```python
from build123d import *

# Parameters (mm, degrees)
BOSS_EXTRUDE1_DEPTH = 10
SKETCH2_R           = 4.05
SKETCH2_R_2         = 1.975
CUT_EXTRUDE1_DEPTH  = 49.845189118
SKETCH14_W          = 50.25
SKETCH14_H          = 4.1
CUT_EXTRUDE13_DEPTH = 5
SKETCH16_W          = 4.6
SKETCH16_H          = 15
CUT_EXTRUDE15_DEPTH = 10
CUT_EXTRUDE14_DEPTH = 49.845189118
SKETCH19_W          = 7
SKETCH19_H          = 5
BOSS_EXTRUDE2_DEPTH = 1
CUT_EXTRUDE16_DEPTH = 8.95
FILLET1_R           = 0.5


with BuildPart() as part:
    # Sketch1 → Boss-Extrude1 (new body)
    with BuildSketch(Plane(origin=(0, 0, 0), x_dir=(1, 0, 0), z_dir=(0, 1, 0))):
        Polygon((-23, 23.2), (23, 23.2), (39.25, 23.2), (39.25, -23.2), (23, -23.2), (23, -27.3), (16, -27.3), (16, -23.2), (3.5, -23.2), (3.5, -27.3), (-3.5, -27.3), (-3.5, -23.2), (-16, -23.2), (-16, -27.3), (-23, -27.3), (-23, -23.2), (-27.25, -23.2), (-27.25, 23.2), align=None)
    extrude(amount=BOSS_EXTRUDE1_DEPTH)

    # Sketch2 → Cut-Extrude1 (cut, through all)
    with BuildSketch(Plane(origin=(0, 10, 0), x_dir=(1, 0, 0), z_dir=(0, 1, 0))):
        with Locations(Location((0, 0, 0), (0, 0, 270))):
            Circle(SKETCH2_R)
        with Locations(Location((-2.025, 15, 0), (0, 0, 270))):
            Circle(SKETCH2_R_2)
        with Locations(Location((-2.025, -15, 0), (0, 0, 270))):
            Circle(SKETCH2_R_2)
    extrude(amount=-CUT_EXTRUDE1_DEPTH, mode=Mode.SUBTRACT)

    # Sketch14 → Cut-Extrude13 (cut)
    with BuildSketch(Plane(origin=(0, 10, 0), x_dir=(1, 0, 0), z_dir=(0, 1, 0))):
        with Locations((-2.125, -25.25)):
            Rectangle(SKETCH14_W, SKETCH14_H)
    extrude(amount=-CUT_EXTRUDE13_DEPTH, mode=Mode.SUBTRACT)

    # Sketch16 → Cut-Extrude15 (cut)
    with BuildSketch(Plane.XZ):
        with Locations((34.45, 0)):
            Rectangle(SKETCH16_W, SKETCH16_H)
        with Locations((-22.45, 0)):
            Rectangle(SKETCH16_W, SKETCH16_H)
    extrude(amount=-CUT_EXTRUDE15_DEPTH, mode=Mode.SUBTRACT)

    # Sketch15 → Cut-Extrude14 (cut, through all)
    with BuildSketch(Plane(origin=(0, 10, 0), x_dir=(1, 0, 0), z_dir=(0, 1, 0))):
        with BuildLine():
            Line((13, -27.3), (13, -23.2))
            ThreePointArc((13, -23.2), (14.5, -21.7), (16, -23.2))
            Line((16, -23.2), (16, -27.3))
            ThreePointArc((16, -27.3), (14.5, -28.8), (13, -27.3))
        make_face()
        with BuildLine():
            Line((3.5, -27.3), (3.5, -23.2))
            ThreePointArc((3.5, -23.2), (5, -21.7), (6.5, -23.2))
            Line((6.5, -23.2), (6.5, -27.3))
            ThreePointArc((6.5, -27.3), (5, -28.8), (3.5, -27.3))
        make_face()
        with BuildLine():
            Line((-13, -27.3), (-13, -23.2))
            ThreePointArc((-13, -23.2), (-14.5, -21.7), (-16, -23.2))
            Line((-16, -23.2), (-16, -27.3))
            ThreePointArc((-16, -27.3), (-14.5, -28.8), (-13, -27.3))
        make_face()
        with BuildLine():
            Line((-3.5, -27.3), (-3.5, -23.2))
            ThreePointArc((-3.5, -23.2), (-5, -21.7), (-6.5, -23.2))
            Line((-6.5, -23.2), (-6.5, -27.3))
            ThreePointArc((-6.5, -27.3), (-5, -28.8), (-3.5, -27.3))
        make_face()
        with BuildLine():
            Line((23, -27.3), (23, -23.2))
            ThreePointArc((23, -23.2), (24.5, -21.7), (26, -23.2))
            Line((26, -23.2), (26, -27.3))
            ThreePointArc((26, -27.3), (24.5, -28.8), (23, -27.3))
        make_face()
        with BuildLine():
            Line((-23, -27.3), (-23, -23.2))
            ThreePointArc((-23, -23.2), (-24.5, -21.7), (-26, -23.2))
            Line((-26, -23.2), (-26, -27.3))
            ThreePointArc((-26, -27.3), (-24.5, -28.8), (-23, -27.3))
        make_face()
        with BuildLine():
            ThreePointArc((34.45, 7.284346805), (31.710660172, 6.439339828), (34.45, 5.594332852))
            ThreePointArc((34.45, 5.594332852), (37.189339828, 6.439339828), (34.45, 7.284346805))
        make_face()
        with BuildLine():
            ThreePointArc((34.45, -7.284346805), (31.710660172, -6.439339828), (34.45, -5.594332852))
            ThreePointArc((34.45, -5.594332852), (37.189339828, -6.439339828), (34.45, -7.284346805))
        make_face()
        with BuildLine():
            ThreePointArc((-22.45, -7.284346805), (-19.710660172, -6.439339828), (-22.45, -5.594332852))
            ThreePointArc((-22.45, -5.594332852), (-25.189339828, -6.439339828), (-22.45, -7.284346805))
        make_face()
        with BuildLine():
            ThreePointArc((-22.45, 7.284346805), (-25.189339828, 6.439339828), (-22.45, 5.594332852))
            ThreePointArc((-22.45, 5.594332852), (-19.710660172, 6.439339828), (-22.45, 7.284346805))
        make_face()
    extrude(amount=-CUT_EXTRUDE14_DEPTH, mode=Mode.SUBTRACT)

    # Sketch19 → Boss-Extrude2 (add)
    with BuildSketch(Plane(origin=(0, 0, -23.2), x_dir=(-1, 0, 0), z_dir=(0, 0, -1))):
        with Locations((-23.83, 2.5)):
            Rectangle(SKETCH19_W, SKETCH19_H)
    extrude(amount=BOSS_EXTRUDE2_DEPTH)

    # Sketch17 → Cut-Extrude16 (cut)
    with BuildSketch(Plane(origin=(0, 10, 0), x_dir=(1, 0, 0), z_dir=(0, 1, 0))):
        with BuildLine():
            Line((25.48, 24.2), (25.48, 15.85))
            ThreePointArc((25.48, 15.85), (23.83, 14.2), (22.18, 15.85))
            Line((22.18, 15.85), (22.18, 24.2))
            ThreePointArc((22.18, 24.2), (23.83, 25.85), (25.48, 24.2))
        make_face()
        with BuildLine():
            Line((1.65, -18.95), (1.65, -27.3))
            ThreePointArc((1.65, -27.3), (0, -28.95), (-1.65, -27.3))
            Line((-1.65, -27.3), (-1.65, -18.95))
            ThreePointArc((-1.65, -18.95), (0, -17.3), (1.65, -18.95))
        make_face()
    extrude(amount=-CUT_EXTRUDE16_DEPTH, mode=Mode.SUBTRACT)

    # Fillet1
    fillet1_edges = [part.edges().sort_by_distance(p)[0] for p in [
        (-27.25, 5, 23.2),
        (-27.25, 5, -23.2),
        (39.25, 5, -23.2),
        (39.25, 5, 23.2),
        (20.33, 2.5, -24.2),
        (27.33, 2.5, -24.2),
        (25.48, 3.025, -24.2),
        (22.18, 3.025, -24.2),
        (-1.65, 3.025, 27.3),
        (1.65, 3.025, 27.3),
        (-16, 2.5, 27.3),
        (-23, 2.5, 27.3),
        (23, 2.5, 27.3),
        (16, 2.5, 27.3),
        (3.5, 2.5, 27.3),
        (-3.5, 2.5, 27.3),
    ]]
    fillet(fillet1_edges, radius=FILLET1_R)


solid = part.part
```
Geometry check sheet. Reference: the model listing, model coordinates, mm. A direction names the side the tool comes from. Coordinates: 2 decimals unless noted, no trailing zeros. Order: outer loops, then holes, each group sorted by start corner. A loop starts at its lowest first (then second) coordinate and runs counter-clockwise, first axis right, second up. Notation, with made-up numbers: M -37,75.5 L -10,75.5 A11 cw -10,89.5 Z; hole C 40,37 d7. An arc over 180 degrees is marked long. Answer as a JSON object with one key per item and string values.
Q1. Cross-section at C-C on x = -5. Record the cut outline in (y, z), and give its area (3 significant figures).
Results are:
{"outline": "M 0,-23.2 L 10,-23.2 L 10,21.7 L 0,21.7 Z", "area": "449 mm²"}
Q2. Depth check by flat-ended pin: pin 1 Ø1.2 at (x, z) = (19, 24.5) entering from +Y; pin 2 Ø2.5 at (x, y) = (19.5, 7.5) entering from +Z; pin 3 Ø3 at (x, z) = (1.5, 10.5) entering from -Y; pin 4 Ø3 at (x, y) = (-2, 5) entering from -Z. Enter the tip coordinate at first touch or a pass-through.
Results are:
{"pin 1": "stops at y = 5", "pin 2": "stops at z = 23.2", "pin 3": "stops at y = 0", "pin 4": "stops at z = -23.2"}
Q3. Scan lines: line 1 (X direction, y = 5, z = 0); line 2 (X direction, y = 2.75, z = 15); line 3 (X direction, y = 4, z = 23.5). Record each from-to range of solid material in increasing order.
Results are:
{"line 1": "x = -27.25 to -24.75, -20.15 to -4.05, 4.05 to 32.15, 36.75 to 39.25", "line 2": "x = -27.25 to -4, -0.05 to 39.25", "line 3": "x = -23 to -16, -3.5 to -1.65, 1.65 to 3.5, 16 to 23"}
Q4. Cross-section at D-D on y = 8. Give the number of separate pieces and of enclosed holes in the cut face, and give its area (3 significant figures).
Results are:
{"separate pieces": "1", "enclosed holes": "5", "area": "2,790 mm²"}
Q5. Cross-section at B-B on z = 0. Record the cut outline in (x, y), and give its area (3 significant figures).
Results are:
{"outline": "M -27.25,0 L -24.75,0 L -24.75,10 L -27.25,10 Z; M -20.15,0 L -4.05,0 L -4.05,10 L -20.15,10 Z; M 4.05,0 L 32.15,0 L 32.15,10 L 4.05,10 Z; M 36.75,0 L 39.25,0 L 39.25,10 L 36.75,10 Z", "area": "492 mm²"}
Q6. Tool access check on faces 4 (the flat face through (32.15, 5, 0)), 5 (the flat face through (3.5, 2, 25)), 6 (the flat face through (-23, 2, 25)), 7 (the cylindrical face through (0, 5.6, 17.3)), 8 (the flat face through (19, 5, 25)). Record the directions out of +Z, -Z, +X, -X, +Y, -Y that give a thin tool (end or side, any length) a straight path to the whole face; none if there is none.
Results are:
{"face 4": "+Y, -Y", "face 5": "+Z, +Y, -Y", "face 6": "+Z, -X, +Y, -Y", "face 7": "+Z, +Y", "face 8": "+Z, +X, -X, +Y"}
Q7. Release check for a two-part mould opening along Z. For faces 1 (the flat face through (-20.15, 5, 0)), 2 (the flat face through (23.9, 0.9, -24.2)), 3 (the flat face through (0, 0.8, 27.3)) record: released by +Z, released by -Z, zero draft, split by the parting line, or undercut.
Results are:
{"face 1": "undercut", "face 2": "released by -Z", "face 3": "released by +Z"}
Q8. Cross-section at A-A on z = 15. Record the cut outline in (x, y), and give its area (4 significant figures).
Results are:
{"outline": "M -27.25,0 L -4,0 L -4,10 L -27.25,10 Z; M -0.05,0 L 39.25,0 L 39.25,10 L -0.05,10 Z", "area": "625.5 mm²"}
